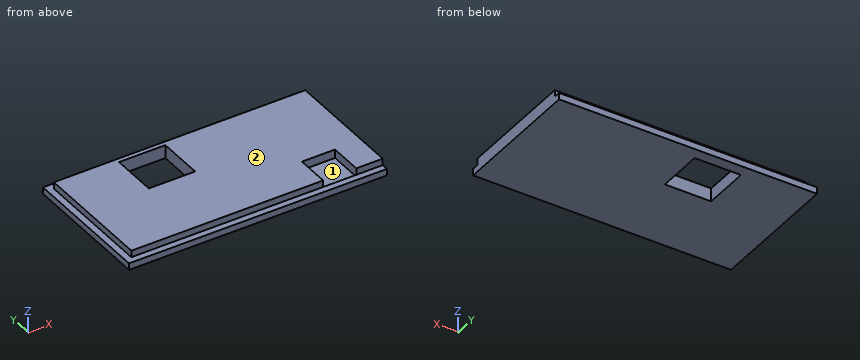
```python
from build123d import *

# Parameters (mm, degrees)
SKETCH1_W           = 39
SKETCH1_H           = 20.2
BOSS_EXTRUDE1_DEPTH = 1
SKETCH2_W           = 38
SKETCH2_H           = 18.2
BOSS_EXTRUDE2_DEPTH = 1
SKETCH3_W           = 7
SKETCH3_H           = 7
CUT_EXTRUDE1_DEPTH  = 21
SKETCH4_W           = 5
SKETCH4_H           = 5
CUT_EXTRUDE2_DEPTH  = 1.3


with BuildPart() as part:
    # Sketch1 → Boss-Extrude1 (new body)
    with BuildSketch(Plane.XY):
        Rectangle(SKETCH1_W, SKETCH1_H)
    extrude(amount=BOSS_EXTRUDE1_DEPTH)

    # Sketch2 → Boss-Extrude2 (add)
    with BuildSketch(Plane.XY.offset(1)):
        with Locations((0.5, 0)):
            Rectangle(SKETCH2_W, SKETCH2_H)
    extrude(amount=BOSS_EXTRUDE2_DEPTH)

    # Sketch3 → Cut-Extrude1 (cut)
    with BuildSketch(Plane.XY.offset(2)):
        with Locations((-5.6, 4.9)):
            Rectangle(SKETCH3_W, SKETCH3_H)
    extrude(amount=-CUT_EXTRUDE1_DEPTH, mode=Mode.SUBTRACT)

    # Sketch4 → Cut-Extrude2 (cut)
    with BuildSketch(Plane.XY.offset(2)):
        with Locations((13, -6.6)):
            Rectangle(SKETCH4_W, SKETCH4_H)
    extrude(amount=-CUT_EXTRUDE2_DEPTH, mode=Mode.SUBTRACT)


solid = part.part
```
Build history of the part. All positions in model axes, mm. Face numbers are marked on the shaded views. Give positions to 0.01 mm unless a question says otherwise; leave off trailing zeros. Order: outer loops, then holes, each group sorted by start corner. A loop starts at its lowest first (then second) coordinate and runs counter-clockwise, first axis right, second up. Notation, with made-up numbers: M 41.25,58.25 L 47.25,58.25 A18 ccw 47.25,87.25 Z; hole C 35,24.25 d3. An arc over 180 degrees is marked long. Return JSON: item names as keys, results as strings.
Q1. Band-saw the part on D-D (x = 13). Give the cut face in (y, z), then the cut area to 3 significant figures.
Answer list:
{"outline": "M -10.1,0 L 10.1,0 L 10.1,1 L 9.1,1 L 9.1,2 L -4.1,2 L -4.1,0.7 L -9.1,0.7 L -9.1,1 L -10.1,1 Z", "area": "31.9 mm^2"}
Q2. Two-plate mould, pull along Y, no slides. Class the marked faces 1 and 2: pulls with the +Y half, pulls with the -Y half, needs draft (parallel to the pull), parting line crosses it, or undercut.
Answer list:
{"face 1": "undercut", "face 2": "needs draft"}
Q3. Band-saw the part on C-C (z = 1.4). Give the cut face in (x, y), then the cut area to 3 significant figures.
Answer list:
{"outline": "M -18.5,-9.1 L 10.5,-9.1 L 10.5,-4.1 L 15.5,-4.1 L 15.5,-9.1 L 19.5,-9.1 L 19.5,9.1 L -18.5,9.1 Z; hole M -9.1,1.4 L -2.1,1.4 L -2.1,8.4 L -9.1,8.4 Z", "area": "618 mm^2"}
Q4. Flat gauge pin, fed straight in: pin 1 (0.6 mm diameter, centred on y = -7.5, z = 1.5, fed in from -X). Where does the tip first touch, or does it go through?
Answer list:
{"pin 1": "stops at x = -18.5"}
Q5. Band-saw the part on A-A (y = 8). Give the cut face in (x, z).
Answer list:
{"outline": "M -19.5,0 L -9.1,0 L -9.1,2 L -18.5,2 L -18.5,1 L -19.5,1 Z; M -2.1,0 L 19.5,0 L 19.5,2 L -2.1,2 Z"}
Q6. Band-saw the part on B-B (x = -4). Give the cut face in (y, z).
Answer list:
{"outline": "M -10.1,0 L 1.4,0 L 1.4,2 L -9.1,2 L -9.1,1 L -10.1,1 Z; M 8.4,0 L 10.1,0 L 10.1,1 L 9.1,1 L 9.1,2 L 8.4,2 Z"}
Q7. Wall check: probe 1 along X at (y, z) = (6.5, 1.6); probe 2 along Y at (x, z) = (-6, 0.3); probe 3 along X at (y, z) = (-4.5, 0.95). Give the ranges that are in metal, low to high. Write a range as from..to.
Answer list:
{"probe 1": "x = -18.5..-9.1, -2.1..19.5", "probe 2": "y = -10.1..1.4, 8.4..10.1", "probe 3": "x = -19.5..10.5, 15.5..19.5"}
